```python
from build123d import *

# Parameters (mm, degrees)
BOSS_EXTRUDE1_DEPTH = 10
FILLET1_R           = 20
CUT_EXTRUDE1_START  = 10
SKETCH2_R           = 11.05
CUT_EXTRUDE1_DEPTH  = 7.3
SKETCH5_R           = 4.15
CUT_EXTRUDE2_DEPTH  = 10
FILLET2_R           = 2
CUT_EXTRUDE3_START  = 4
SKETCH6_R           = 4
CUT_EXTRUDE3_DEPTH  = 13
SKETCH7_R           = 2
CUT_EXTRUDE4_DEPTH  = 13
CUT_EXTRUDE5_START  = 10
SKETCH9_R           = 1.5
CUT_EXTRUDE5_DEPTH  = 7.5


with BuildPart() as part:
    # Sketch1 → Boss-Extrude1 (new body)
    with BuildSketch(Plane.XY):
        with BuildLine():
            Line((0, 12), (18.029437252, 12))
            ThreePointArc((18.029437252, 12), (35, 36), (51.970562748, 12))
            Line((51.970562748, 12), (70, 12))
            Line((70, 12), (70, 0))
            Line((70, 0), (0, 0))
            Line((0, 0), (0, 12))
        make_face()
    extrude(amount=BOSS_EXTRUDE1_DEPTH)

    # Fillet1
    # the kernel refuses this fillet: 20 mm, written as the material it adds along each edge
    with BuildSketch(Plane(origin=(18.029437252, 12, 0), x_dir=(-1, 0, 0), z_dir=(0, 0, 1))) as fillet1_piece_1:
        with BuildLine():
            CenterArc((18.357547265, -19.997308414), FILLET1_R, 90.94000812, 67.446084787)
            Line((-0.236194847, -12.630303986), (-0.608069689, -12.482963897))
            ThreePointArc((-0.608069689, -12.482963897), (0.626360574, -6.329073839), (-0.377123617, -0.133333333))
            Line((-0.377123617, -0.133333333), (0, 0.4))
            ThreePointArc((0, 0.4), (9.014718626, 0.4), (18.022875051, 0.399946168))
            Line((18.022875051, 0.399946168), (18.029437252, 0))
        make_face()
    extrude(amount=10)
    with BuildSketch(Plane(origin=(51.970562748, 12, 0), x_dir=(-0.018697377190164018, 0.9998251887636201, 0), z_dir=(0, 0, 1))) as fillet1_piece_2:
        with BuildLine():
            CenterArc((19.650574675, -18.728235378), FILLET1_R, 110.542563864, 67.446084787)
            Line((-0.337103189, -18.026285503), (-0.736856746, -18.012246506))
            ThreePointArc((-0.736856746, -18.012246506), (-0.56848167, -9.005663801), (-0.399930076, 0.007478951))
            Line((-0.399930076, 0.007478951), (0.140361248, 0.374564708))
            ThreePointArc((0.140361248, 0.374564708), (6.316256145, -0.74458816), (12.492151043, 0.374564708))
            Line((12.492151043, 0.374564708), (12.632512291, 0))
        make_face()
    extrude(amount=10)

    # Sketch2 → Cut-Extrude1 (cut)
    with BuildSketch(Plane.XY.offset(CUT_EXTRUDE1_START)):
        with Locations(Location((35, 18, 0), (0, 0, 180))):
            Circle(SKETCH2_R)
    extrude(amount=-CUT_EXTRUDE1_DEPTH, mode=Mode.SUBTRACT)

    # Sketch5 → Cut-Extrude2 (cut)
    with BuildSketch(Plane.XY):
        with Locations(Location((35, 18, 0), (0, 0, 180))):
            Circle(SKETCH5_R)
    extrude(amount=CUT_EXTRUDE2_DEPTH, mode=Mode.SUBTRACT)

    # Fillet2
    fillet2_edges = [part.edges().sort_by_distance(p)[0] for p in [
        (0, 12, 5),
        (70, 12, 5),
    ]]
    fillet(fillet2_edges, radius=FILLET2_R)

    # Sketch6 → Cut-Extrude3 (cut)
    with BuildSketch(Plane(origin=(0, 0, 0), x_dir=(1, 0, 0), z_dir=(0, 1, 0)).offset(CUT_EXTRUDE3_START)):
        with Locations(Location((8, -5, 0), (0, 0, 90))):
            Circle(SKETCH6_R)
        with Locations(Location((62, -5, 0), (0, 0, 90))):
            Circle(SKETCH6_R)
    extrude(amount=CUT_EXTRUDE3_DEPTH, mode=Mode.SUBTRACT)

    # Sketch7 → Cut-Extrude4 (cut)
    with BuildSketch(Plane(origin=(0, 0, 0), x_dir=(1, 0, 0), z_dir=(0, 1, 0))):
        with Locations(Location((8, -5, 0), (0, 0, 90))):
            Circle(SKETCH7_R)
        with Locations(Location((62, -5, 0), (0, 0, 90))):
            Circle(SKETCH7_R)
    extrude(amount=CUT_EXTRUDE4_DEPTH, mode=Mode.SUBTRACT)

    # Sketch9 → Cut-Extrude5 (cut)
    with BuildSketch(Plane.XY.offset(CUT_EXTRUDE5_START)):
        with Locations(Location((20, 18, 0), (0, 0, 180))):
            Circle(SKETCH9_R)
        with Locations(Location((50, 18, 0), (0, 0, 180))):
            Circle(SKETCH9_R)
    extrude(amount=-CUT_EXTRUDE5_DEPTH, mode=Mode.SUBTRACT)


solid = part.part
```
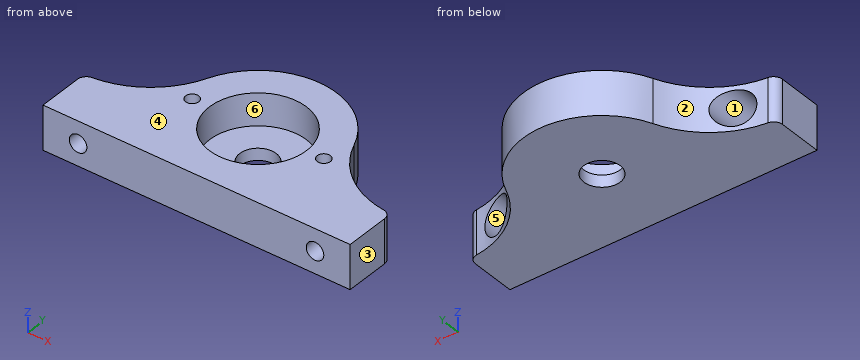
Geometry check sheet. Reference: the model listing, model coordinates, mm. Face numbers are marked on the shaded views. A direction names the side the tool comes from. Coordinates: 2 decimals unless noted, no trailing zeros. Order: outer loops, then holes, each group sorted by start corner. A loop starts at its lowest first (then second) coordinate and runs counter-clockwise, first axis right, second up. Notation, with made-up numbers: (39, -23) - (65, -23) arc R18 ccw to (65, 2) - close; hole circle Ø6 at (74.25, 32). An arc over 180 degrees is marked (long way). Answer in a Markdown table with one row per item. Add a question column.
1. Access from +Z, -Z, +X, -X, +Y, -Y to the whole of each face (thin tool, end or side, straight path). Record for the marked faces 4, 5 and 6.
2. Section check C-C (y = 18). Enter the section's corners in (x, z), plus the area to 3 significant figures.
3. Draft check along X on the marked faces 1, 2 and 3. Enter one of: +X half, -X half, draft (parallel to the pull), parting line (faces both ways), or undercut.
4. Gauge pin test, flat ends, axial feed: pin 1 Ø1.5 at (x, z) = (16.5, 8.5) entering from +Y; pin 2 Ø2.5 at (x, z) = (9.5, 4.5) entering from +Y; pin 3 Ø1 at (y, z) = (15.5, 5) entering from +X. Record the tip position at first contact, or that the pin passes through.
5. Section check B-B (z = 6.25). Enter the section's corners in (x, y).
6. Material ranges on L1, parallel to X at y = 1, z = 5; L2, parallel to X at y = 18, z = 6.25; L3, parallel to Y at x = 35, z = 1.3, recorded low to high. Write a range as [from, to].
7. Section check D-D (y = 8.5). Enter the section's corners in (x, z).
8. Section check A-A (x = 35). Enter the section's corners in (y, z).
Data:
| question | item | result |
|---|---|---|
| 1 | face 4 | +Z, +X, -X, +Y, -Y |
| 1 | face 5 | +Y |
| 1 | face 6 | +Z |
| 2 | outline | (13.96, 0) - (30.85, 0) - (30.85, 2.7) - (23.95, 2.7) - (23.95, 10) - (21.5, 10) - (21.5, 2.5) - (18.5, 2.5) - (18.5, 10) - (13.96, 10) - close; (39.15, 0) - (56.04, 0) - (56.04, 10) - (51.5, 10) - (51.5, 2.5) - (48.5, 2.5) - (48.5, 10) - (46.05, 10) - (46.05, 2.7) - (39.15, 2.7) - close |
| 2 | area | 192 mm² |
| 3 | face 1 | undercut |
| 3 | face 2 | -X half |
| 3 | face 3 | +X half |
| 4 | pin 1 | stops at y = 22.46 |
| 4 | pin 2 | stops at y = 4 |
| 4 | pin 3 | stops at x = 58.03 |
| 5 | outline | (0, 0) - (6.44, 0) - (6.44, 4) - (4.2, 4) - (4.2, 12.52) arc R20 cw to (1.79, 12.11) arc R2 ccw to (0, 10.12) - close; (9.56, 0) - (60.44, 0) - (60.44, 4) - (58.2, 4) - (58.2, 16.09) arc R20 cw to (51.73, 24.63) arc R18 ccw to (18.27, 24.63) arc R20 cw to (11.8, 16.09) - (11.8, 4) - (9.56, 4) - close; (63.56, 0) - (70, 0) - (70, 10.12) arc R2 ccw to (68.21, 12.11) arc R20 cw to (65.8, 12.52) - (65.8, 4) - (63.56, 4) - close; hole circle Ø3 at (20, 18); hole circle Ø22.1 at (35, 18); hole circle Ø3 at (50, 18) |
| 6 | L1 | x = [0, 6], [10, 60], [64, 70] |
| 6 | L2 | x = [13.96, 18.5], [21.5, 23.95], [46.05, 48.5], [51.5, 56.04] |
| 6 | L3 | y = [0, 13.85], [22.15, 36] |
| 7 | outline | (0, 0) - (70, 0) - (70, 10) - (40.64, 10) - (40.64, 2.7) - (29.36, 2.7) - (29.36, 10) - (0, 10) - close; hole circle Ø8 at (8, 5); hole circle Ø8 at (62, 5) |
| 8 | outline | (0, 0) - (13.85, 0) - (13.85, 2.7) - (6.95, 2.7) - (6.95, 10) - (0, 10) - close; (22.15, 0) - (36, 0) - (36, 10) - (29.05, 10) - (29.05, 2.7) - (22.15, 2.7) - close |
